```python
from build123d import *

# Parameters (mm, degrees)
F0_W     = 1.5
F0_H     = 2.5
F0_W_2   = 84
F0_H_2   = 5
F0_W_3   = 6
F0_H_3   = 1.23
F0_H_4   = 0.27
F3_DEPTH = 32
F4_W     = 10
F4_H     = 1
F5_DEPTH = 12.5
F8_D     = 3
F8_DEPTH = 6
F8_TIP   = 0.9012909285


# Not quite as in the source:
# - ends of sketch curves that miss each other by under 0.0002 mm in the source are joined


with BuildPart() as f1:
    # F0 (on Front) → F1 (revolve)
    with BuildSketch(Plane.XZ):
        with Locations((0.75, 1.25)):
            Rectangle(F0_W, F0_H)
        Polygon((-10, 0), (-5, 0), (-5, 4.123106), align=None)
        Polygon((-8.210141, 6), (-7.5, 6), (-7.5, 7.23), align=None)
        Polygon((-15, 0), (-10, 0), (-15, 4.123106), align=None)
        with Locations((-62, 2.5)):
            Rectangle(F0_W_2, F0_H_2)
        Polygon((0, 0), (0, 2.5), (0, 4.5), (-6, 4.5), (-6.467654, 4.77), (-7.5, 4.77), (-8.210141, 6), (-7.5, 7.23), (-6.467654, 7.23), (-6, 7.5), (0, 7.5), (0, 9), (-20, 9), (-20, 5), (-20, 0), (-15, 0), (-15, 4.123106), (-5, 4.123106), (-5, 0), align=None)
        Polygon((-15, 4.123106), (-9.9999998364, 3.651e-07), (-5, 4.123106), align=None)
        with Locations((-3, 6.615)):
            Rectangle(F0_W_3, F0_H_3)
        Polygon((2, 2), (1.5, 2.5), (1.5, 0), (2, 0), align=None)
        with Locations((-3, 5.385)):
            Rectangle(F0_W_3, F0_H_3)
        Polygon((-7.5, 6), (-6, 6), (-6, 7.23), (-6.467654, 7.23), (-7.5, 7.23), align=None)
        Polygon((-6.467654, 4.77), (-6, 4.77), (-6, 6), (-7.5, 6), (-7.5, 4.77), align=None)
        Polygon((-8.210141, 6), (-7.5, 4.77), (-7.5, 6), align=None)
        with Locations((-3, 7.365)):
            Rectangle(F0_W_3, F0_H_4)
        with Locations((-3, 4.635)):
            Rectangle(F0_W_3, F0_H_4)
        Polygon((-6.467654, 4.77), (-6, 4.5), (-6, 4.77), align=None)
        Polygon((-6.467654, 7.23), (-6, 7.23), (-6, 7.5), align=None)
        Polygon((-105, 0), (-104, 0), (-104, 5), (-105, 4), align=None)
    revolve(axis=Axis((-53, 0, 0), (-1, 0, 0)))

    # F2 (on face) → F3 (cut)
    with BuildSketch(Plane(origin=(-105, 0, 0), x_dir=(0, -1, 0), z_dir=(-1, 0, 0))):
        with BuildLine():
            Line((-3.1224989992, -2.5), (-4.330127, -2.5))
            ThreePointArc((-4.3301270142, -2.5000000082), (0, -5), (4.3301270142, -2.5000000082))
            Line((4.330127, -2.5), (3.1224989992, -2.5))
            ThreePointArc((3.1224989992, -2.5), (0, -4), (-3.1224989992, -2.5))
        make_face()
        with BuildLine():
            Line((3.1224989992, -2.5), (-3.1224989992, -2.5))
            ThreePointArc((-3.1224989992, -2.5), (0, -4), (3.1224989992, -2.5))
        make_face()
    extrude(amount=-F3_DEPTH, mode=Mode.SUBTRACT)

    # F4 (on Top) → F5 (cut, symmetric)
    with BuildSketch(Plane.XY):
        with Locations((-10, -8.5)):
            Rectangle(F4_W, F4_H)
        with Locations((-10, 8.5)):
            Rectangle(F4_W, F4_H)
    extrude(amount=F5_DEPTH, both=True, mode=Mode.SUBTRACT)

    # F8
    with Locations(Plane.YZ):
        with Locations((0, 6), (1.552915, -5.795555)):
            Hole(F8_D / 2, depth=F8_DEPTH)
            with Locations((0, 0, -(F8_DEPTH + F8_TIP / 2))):  # 118° drill point
                Cone(0, F8_D / 2, F8_TIP, mode=Mode.SUBTRACT)


solid = f1.part
```
The model under review builds one solid part; all positions refer to its coordinate system, in mm. A direction names the side the tool comes from. Round coordinates to 2 decimals unless told otherwise and drop trailing zeros. Loops run counter-clockwise (first coordinate to the right, second up) from the corner with the lowest first, then second, coordinate; pieces in that order, holes last. Notation, with made-up numbers: (-16, -18) -> (1, -18) arc R24 cw to (1, 4) -> close; hole circle Ø3 at (49.25, 58.5). An arc over 180 degrees is marked (long way). Answer as a JSON object with one key per item and string values. Group by question number.
1) Mouldability with a two-part tool opening along Z and no side actions: class faces 5 (the face through (-104.8, -0.1, 4.2)), 6 (the face through (-6.745, 0.12, 5.769)), 7 (the face through (-105, 0, 1)), 8 (the face through (-89, 0, -2.5)) as released by +Z, released by -Z, zero draft, split by the parting line, or undercut.
2) We need section D-D on x = -28.5. Write out the cut boundary in (y, z).
3) We need section B-B on x = -80. Write out the cut boundary in (y, z).
4) We need section C-C on y = 6.5. Write out the cut boundary in (x, z).
5) For line 1 (Y direction, x = -70.5, z = -0.25); line 2 (X direction, y = -6.5, z = -1.75); line 3 (Y direction, x = -4.75, z = 6), list the stretches that pass through material, from the lowest coordinate up. Write a range as [from, to].
6) We need section A-A on z = 0. Write out the cut boundary in (x, y).
7) For pin 1 Ø1.8 at (y, z) = (0, 6) entering from +X; pin 2 Ø4 at (x, z) = (-10.5, 1) entering from +Y; pin 3 Ø1.1 at (y, z) = (8.5, -1) entering from -X, all flat-tipped, find the tip position at first contact; note any pin that passes through.
8) For faces 1 (the face through (-73, 0, -3)), 2 (the face through (-10, -8, 0)), 3 (the face through (-61.41, 1.5, 4.77)), 4 (the face through (-3.04, 1.88, -7.26)), list the 3-axis set-ups (+Z, -Z, +X, -X, +Y, -Y) from which the entire face can be reached by the end or side of a thin tool; tool diameter is ignored.
Result set:
{
 "1": {"face 5": "split by the parting line", "face 6": "undercut", "face 7": "zero draft", "face 8": "released by -Z"},
 "2": {"outline": "circle Ø10 at (0, 0)"},
 "3": {"outline": "(-4.33, -2.5) -> (4.33, -2.5) arc R5 ccw (long way) to start"},
 "4": {"outline": "(-20, -6.22) -> (0, -6.22) -> (0, 6.22) -> (-20, 6.22) -> close"},
 "5": {"line 1": "[-4.99, 4.99]", "line 2": "[-20, 0]", "line 3": "[-6.71, -1.5], [1.5, 6.71]"},
 "6": {"outline": "(-105, -4) -> (-104, -5) -> (-20, -5) -> (-20, -9) -> (-15, -9) -> (-15, -8) -> (-5, -8) -> (-5, -9) -> (0, -9) -> (0, -2.5) -> (1.5, -2.5) -> (2, -2) -> (2, 2) -> (1.5, 2.5) -> (0, 2.5) -> (0, 9) -> (-5, 9) -> (-5, 8) -> (-15, 8) -> (-15, 9) -> (-20, 9) -> (-20, 5) -> (-104, 5) -> (-105, 4) -> close"},
 "7": {"pin 1": "x = -6.36", "pin 2": "y = 8", "pin 3": "x = -20"},
 "8": {"face 1": "-Z, -X, +Y, -Y", "face 2": "+Z, -Z, -Y", "face 3": "-X", "face 4": "+X"}
}
